```python
from build123d import *

# Parameters (mm, degrees)
CUT_EXTRUDE1_DEPTH = 2.286


with BuildPart() as part:
    # Sketch1 → Revolve1 (revolve)
    with BuildSketch(Plane.XY):
        Polygon((0, 2.413), (0, 3.5814), (-0.381, 3.9624), (-4.445, 3.9624), (-4.826, 3.5814), (-4.826, 2.291358881), (-2.534641119, 0), (19.05, 0), (19.05, 1.651), (18.288, 2.413), align=None)
    revolve(axis=Axis((-2.534641119, 0, 0), (-1, 0, 0)))

    # Sketch2 → Cut-Extrude1 (cut)
    with BuildSketch(Plane.ZY.offset(4.826)):
        Polygon((0, 2.291358881), (-1.984375, 1.14567944), (-1.984375, -1.14567944), (0, -2.291358881), (1.984375, -1.14567944), (1.984375, 1.14567944), align=None)
    extrude(amount=-CUT_EXTRUDE1_DEPTH, mode=Mode.SUBTRACT)


solid = part.part
```
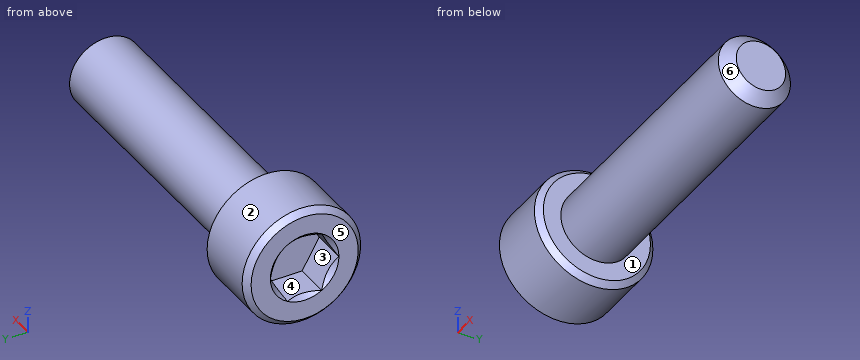
Geometry check sheet. Reference: the model listing, model coordinates, mm. Face numbers are marked on the shaded views. A direction names the side the tool comes from. Coordinates: 2 decimals unless noted, no trailing zeros. Order: outer loops, then holes, each group sorted by start corner. A loop starts at its lowest first (then second) coordinate and runs counter-clockwise, first axis right, second up. Notation, with made-up numbers: (61.25, 79.25) - (119.25, 79.25) arc R21 ccw to (119.25, 89.25) - close; hole circle Ø7 at (83, 76.5). An arc over 180 degrees is marked (long way). Answer as a JSON object with one key per item and string values. Group by question number.
Item 1: Depth check by flat-ended pin: pin 1 Ø1 at (y, z) = (3, -1) entering from +X; pin 2 Ø2 at (x, z) = (7, -2.5) entering from -Y; pin 3 Ø0.7 at (x, y) = (-4, 0.5) entering from +Z. Enter the tip coordinate at first touch or a pass-through.
Item 2: Sectioned sample at A-A, the plane x = 11.5. Record the cut outline in (y, z), and give its area (3 significant figures).
Item 3: Scan lines: probe 1 along X at (y, z) = (0.25, 3.5); probe 2 along X at (y, z) = (0.5, -0.5); probe 3 along Y at (x, z) = (8.5, -0.75). Record each from-to range of solid material in increasing order.
Item 4: Tool access check on the marked faces 1, 2 and 3. Record the directions out of +Z, -Z, +X, -X, +Y, -Y that give a thin tool (end or side, any length) a straight path to the whole face; none if there is none.
Item 5: Draft check along Z on the marked faces 4, 5 and 6. Enter one of: +Z half, -Z half, draft (parallel to the pull), parting line (faces both ways), or undercut.
Resolved:
{
 "1": {"pin 1": "x = 0", "pin 2": "y = -1.89", "pin 3": "z = 3.96"},
 "2": {"outline": "circle Ø4.83 at (0, 0)", "area": "18.3 mm^2"},
 "3": {"probe 1": "-4.83 to 0", "probe 2": "-2.54 to 19.05", "probe 3": "-2.29 to 2.29"},
 "4": {"face 1": "+X", "face 2": "+X, -X", "face 3": "-X"},
 "5": {"face 4": "undercut", "face 5": "draft", "face 6": "parting line"}
}
